Geometry check sheet. Reference: the model listing, model coordinates, mm. Give positions to 0.01 mm unless a question says otherwise; leave off trailing zeros. Write each loop counter-clockwise with the first axis right and the second up, starting at its lowest first coordinate (ties: lowest second). Pieces come first, ordered by that corner, then holes. Notation, with made-up numbers: (9.25, 36.5) -> (23.25, 36.5) arc R31 ccw to (23.25, 69.5) -> close; hole circle Ø5 at (28.5, 32.5). An arc over 180 degrees is marked (long way). Write item = value, one per line. Start each with the question number.
1. Cross-section at A-A, the plane z = 92. Record the cut outline in (x, y).
2. Thickness scan on line 1 along X through (y, z) = (90.75, 759.5); line 2 along X through (y, z) = (92.25, 557); line 3 along Y through (x, z) = (9.25, 96). Record the ranges inside material, lowest first.
3. Cross-section at B-B, the plane x = 5.75. Record the cut outline in (y, z), plus the area to 3 significant figures.
4. Depth check by flat-ended pin: P1, Ø1, axis at y = 92.5, z = 698, coming from the -X side; P2, Ø1, axis at y = 90, z = 126.5, coming from the -X side; P3, Ø1.5, axis at y = 90.5, z = 294, coming from the -X side. Enter the tip coordinate at first touch or a pass-through.
```python
from build123d import *

# Parameters (mm, degrees)
EXTRUDE_1_DEPTH = 1000


with BuildPart() as part:
    # 草图1 → 拉伸1 (new body)
    with BuildSketch(Plane.XY):
        with BuildLine():
            Line((9.957625481, 89.483322587), (10.600277657, 91.248994929))
            ThreePointArc((10.600277657, 91.248994929), (10.620053384, 91.338197469), (10.616067953, 91.429478841))
            Line((10.616067953, 91.429478841), (10.013039731, 94.849421835))
            Line((10.013039731, 94.849421835), (3.609954409, 94.849421835))
            Line((3.609954409, 94.849421835), (3.007969074, 91.435393352))
            ThreePointArc((3.007969074, 91.435393352), (3.003983643, 91.34411198), (3.02375937, 91.25490944))
            Line((3.02375937, 91.25490944), (3.665329884, 89.49220894))
            ThreePointArc((3.665329884, 89.49220894), (3.426260893, 88.979523834), (2.913575787, 89.218592825))
            Line((2.913575787, 89.218592825), (2.25631362, 91.024405789))
            ThreePointArc((2.25631362, 91.024405789), (2.199811543, 91.27927019), (2.211198488, 91.54007411))
            Line((2.211198488, 91.54007411), (2.79472578, 94.849421835))
            Line((2.79472578, 94.849421835), (2.11149707, 94.849421835))
            ThreePointArc((2.11149707, 94.849421835), (1.970075714, 94.908000479), (1.91149707, 95.049421835))
            Line((1.91149707, 95.049421835), (1.91149707, 95.349421835))
            ThreePointArc((1.91149707, 95.349421835), (1.999365035, 95.56155387), (2.21149707, 95.649421835))
            Line((2.21149707, 95.649421835), (11.41149707, 95.649421835))
            ThreePointArc((11.41149707, 95.649421835), (11.623629104, 95.56155387), (11.71149707, 95.349421835))
            Line((11.71149707, 95.349421835), (11.71149707, 95.049421835))
            ThreePointArc((11.71149707, 95.049421835), (11.652918426, 94.908000479), (11.51149707, 94.849421835))
            Line((11.51149707, 94.849421835), (10.826662681, 94.849421835))
            Line((10.826662681, 94.849421835), (11.411756877, 91.531187757))
            ThreePointArc((11.411756877, 91.531187757), (11.423143822, 91.270383837), (11.366641745, 91.015519436))
            Line((11.366641745, 91.015519436), (10.709379578, 89.209706473))
            ThreePointArc((10.709379578, 89.209706473), (10.196694472, 88.970637482), (9.957625481, 89.483322587))
        make_face()
    extrude(amount=EXTRUDE_1_DEPTH)


solid = part.part
```
Answers:
q1.outline = (1.91, 95.05) arc R0.2 ccw to (2.11, 94.85) -> (2.79, 94.85) -> (2.21, 91.54) arc R1 ccw to (2.26, 91.02) -> (2.91, 89.22) arc R0.4 ccw to (3.67, 89.49) -> (3.02, 91.25) arc R0.35 cw to (3.01, 91.44) -> (3.61, 94.85) -> (10.01, 94.85) -> (10.62, 91.43) arc R0.35 cw to (10.6, 91.25) -> (9.96, 89.48) arc R0.4 ccw to (10.71, 89.21) -> (11.37, 91.02) arc R1 ccw to (11.41, 91.53) -> (10.83, 94.85) -> (11.51, 94.85) arc R0.2 ccw to (11.71, 95.05) -> (11.71, 95.35) arc R0.3 ccw to (11.41, 95.65) -> (2.21, 95.65) arc R0.3 ccw to (1.91, 95.35) -> close
q2.line_1 = 2.36 to 3.21, 10.42 to 11.27
q2.line_2 = 2.34 to 3.15, 10.47 to 11.29
q2.line_3 = 94.85 to 95.65
q3.outline = (94.85, 0) -> (95.65, 0) -> (95.65, 1000) -> (94.85, 1000) -> close
q3.area = 800 mm^2
q4.P1 = 2.29
q4.P2 = 2.45
q4.P3 = 2.2
